For this review, take the finished solid that the model builds, in its own axes (mm). A direction names the side the tool comes from. Give positions to 0.01 mm unless a question says otherwise; leave off trailing zeros. Order: outer loops, then holes, each group sorted by start corner. A loop starts at its lowest first (then second) coordinate and runs counter-clockwise, first axis right, second up. Notation, with made-up numbers: (-4, 53.25) - (10, 53.25) arc R9 ccw to (10, 63.25) - close; hole circle Ø11 at (-24, 54). An arc over 180 degrees is marked (long way). Answer as a JSON object with one key per item and string values. Group by question number.
from build123d import *

# Parameters (mm, degrees)
SKIZZE1_W                       = 180
SKIZZE1_H                       = 150
AUFSATZ_LINEAR_AUSTRAGEN1_DEPTH = 10
SKIZZE2_W                       = 85
SKIZZE2_H                       = 47
AUFSATZ_LINEAR_AUSTRAGEN2_DEPTH = 5
SKIZZE4_R                       = 2.35
SCHNITT_LINEAR_AUSTRAGEN1_DEPTH = 119.11011811
SKIZZE5_R                       = 4.5
SCHNITT_LINEAR_AUSTRAGEN2_DEPTH = 9


with BuildPart() as part:
    # Skizze1 → Aufsatz-Linear austragen1 (new body)
    with BuildSketch(Plane.XY):
        Rectangle(SKIZZE1_W, SKIZZE1_H)
    extrude(amount=AUFSATZ_LINEAR_AUSTRAGEN1_DEPTH)

    # Skizze2 → Aufsatz-Linear austragen2 (add)
    with BuildSketch(Plane.XY.offset(10)):
        with Locations((0, 38.5)):
            Rectangle(SKIZZE2_W, SKIZZE2_H)
    aufsatz_linear_austragen2 = extrude(amount=AUFSATZ_LINEAR_AUSTRAGEN2_DEPTH)

    # Skizze4 → Schnitt-Linear austragen1 (cut, symmetric)
    with BuildSketch(Plane.XY.offset(15)):
        with Locations((-20, 56.8)):
            Circle(SKIZZE4_R)
        with Locations((-20, 18.2)):
            Circle(SKIZZE4_R)
        with Locations((20, 56.8)):
            Circle(SKIZZE4_R)
        with Locations((20, 18.2)):
            Circle(SKIZZE4_R)
    schnitt_linear_austragen1 = extrude(amount=SCHNITT_LINEAR_AUSTRAGEN1_DEPTH, both=True, mode=Mode.SUBTRACT)

    # Skizze5 → Schnitt-Linear austragen2 (cut)
    with BuildSketch(Plane(origin=(0, 0, 0), x_dir=(-1, 0, 0), z_dir=(0, 0, -1))):
        with Locations((-20, 56.8)):
            Circle(SKIZZE5_R)
        with Locations((20, 56.8)):
            Circle(SKIZZE5_R)
        with Locations((20, 18.2)):
            Circle(SKIZZE5_R)
        with Locations((-20, 18.2)):
            Circle(SKIZZE5_R)
    schnitt_linear_austragen2 = extrude(amount=-SCHNITT_LINEAR_AUSTRAGEN2_DEPTH, mode=Mode.SUBTRACT)

    # Spiegeln8: Aufsatz-Linear austragen2, Schnitt-Linear austragen1, Schnitt-Linear austragen2 across plane
    add(aufsatz_linear_austragen2.mirror(Plane.ZX))
    add(schnitt_linear_austragen1.mirror(Plane.ZX), mode=Mode.SUBTRACT)
    add(schnitt_linear_austragen2.mirror(Plane.ZX), mode=Mode.SUBTRACT)


solid = part.part
1) Consider section D-D (x = -45). Give the boundary of the cut face in (y, z), plus the area to 3 significant figures.
2) For pin 1 (5.5 mm diameter, centred on x = -20, y = -18.2, fed in from -Z); pin 2 (3 mm diameter, centred on x = 51, z = 12, fed in from -Y); pin 3 (5.5 mm diameter, centred on y = -48.5, z = 13, fed in from -X); pin 4 (2 mm diameter, centred on x = 32, z = 12, fed in from +Y), all flat-tipped, find the tip position at first contact; note any pin that passes through.
3) Mouldability with a two-part tool opening along X and no side actions: class faces 1 (the face through (23.6, 15.5, 4.4)), 2 (the face through (-42.5, -38, 12)), 3 (the face through (-1, 1, 10)) as released by +X, released by -X, zero draft, split by the parting line, or undercut.
4) For line 1 (X direction, y = -56.8, z = 12.9); line 2 (Y direction, x = -19.5, z = 1.25); line 3 (X direction, y = -18.2, z = 3.5), list the stretches that pass through material, from the lowest coordinate up.
5) Consider section A-A (z = 12.25). Give the number of separate pieces and of enclosed holes in the cut face, plus the area to 3 significant figures.
6) Consider section B-B (y = -56.8). Give the boundary of the cut face in (x, z), plus the area to 3 significant figures.
7) For faces 4 (the face through (-1, -15, 12)), 5 (the face through (42.5, 38, 12)), 6 (the face through (-22, -16, 9)), list the 3-axis set-ups (+Z, -Z, +X, -X, +Y, -Y) from which the entire face can be reached by the end or side of a thin tool; tool diameter is ignored.
Result set:
{
 "1": {"outline": "(-75, 0) - (75, 0) - (75, 10) - (-75, 10) - close", "area": "1,500 mm2"},
 "2": {"pin 1": "stops at z = 9", "pin 2": "passes through", "pin 3": "stops at x = -42.5", "pin 4": "stops at y = 62"},
 "3": {"face 1": "undercut", "face 2": "released by -X", "face 3": "zero draft"},
 "4": {"line 1": "x = -42.5 to -22.35, -17.65 to 17.65, 22.35 to 42.5", "line 2": "y = -75 to -61.27, -52.33 to -22.67, -13.73 to 13.73, 22.67 to 52.33, 61.27 to 75", "line 3": "x = -90 to -24.5, -15.5 to 15.5, 24.5 to 90"},
 "5": {"separate pieces": "2", "enclosed holes": "8", "area": "7,850 mm2"},
 "6": {"outline": "(-90, 0) - (-24.5, 0) - (-24.5, 9) - (-22.35, 9) - (-22.35, 15) - (-42.5, 15) - (-42.5, 10) - (-90, 10) - close; (-17.65, 9) - (-15.5, 9) - (-15.5, 0) - (15.5, 0) - (15.5, 9) - (17.65, 9) - (17.65, 15) - (-17.65, 15) - close; (22.35, 9) - (24.5, 9) - (24.5, 0) - (90, 0) - (90, 10) - (42.5, 10) - (42.5, 15) - (22.35, 15) - close", "area": "2,010 mm2"},
 "7": {"face 4": "+Z, +X, -X", "face 5": "+Z, +X, +Y, -Y", "face 6": "-Z"}
}
